from build123d import *

# Parameters (mm, degrees)
SKETCH_1_W          = 10
SKETCH_1_H          = 10
SKETCH_1_W_2        = 8
SKETCH_1_H_2        = 8
EXTRUDE_1_DEPTH     = 90
SKETCH_2_R          = 1.5
CUT_EXTRUDE_1_DEPTH = 30
SKETCH_3_R          = 1.5
CUT_EXTRUDE_2_DEPTH = 30


with BuildPart() as part:
    # 草图1 → 凸台-拉伸1 (new body)
    with BuildSketch(Plane(origin=(0, 0, 0), x_dir=(1, 0, 0), z_dir=(0, 1, 0))):
        Rectangle(SKETCH_1_W, SKETCH_1_H)
        Rectangle(SKETCH_1_W_2, SKETCH_1_H_2, mode=Mode.SUBTRACT)
    extrude(amount=EXTRUDE_1_DEPTH)

    # 草图2 → 切除-拉伸1 (cut)
    with BuildSketch(Plane.ZY.offset(5)):
        with Locations((0, 84)):
            Circle(SKETCH_2_R)
        with Locations((0, 74)):
            Circle(SKETCH_2_R)
    extrude(amount=-CUT_EXTRUDE_1_DEPTH, mode=Mode.SUBTRACT)

    # 草图3 → 切除-拉伸2 (cut)
    with BuildSketch(Plane.XY.offset(5)):
        with Locations((0, 5)):
            Circle(SKETCH_3_R)
        with Locations((0, 15)):
            Circle(SKETCH_3_R)
    extrude(amount=-CUT_EXTRUDE_2_DEPTH, mode=Mode.SUBTRACT)


solid = part.part
Read the model definition and answer for the solid it produces. Units are mm, in the model's axes. A direction names the side the tool comes from. Coordinates: 2 decimals unless noted, no trailing zeros. Loops run counter-clockwise (first coordinate to the right, second up) from the corner with the lowest first, then second, coordinate; pieces in that order, holes last. Notation, with made-up numbers: (41.5, 21.5) - (63.5, 21.5) arc R29 cw to (63.5, 43.5) - close; hole circle Ø4 at (35.25, -37). An arc over 180 degrees is marked (long way). Answer in a Markdown table with one row per item.
Q1. Find section B-B on y = 15. Write down the section's boundary in (x, z).
Here are the results:
| item | result |
|---|---|
| outline | (-5, -5) - (-1.5, -5) - (-1.5, -4) - (-4, -4) - (-4, 4) - (-1.5, 4) - (-1.5, 5) - (-5, 5) - close; (1.5, -5) - (5, -5) - (5, 5) - (1.5, 5) - (1.5, 4) - (4, 4) - (4, -4) - (1.5, -4) - close |
Q2. Straight lines are drawn through the part: line 1 along Y through (x, z) = (0, -4.2); line 2 along Y through (x, z) = (-4.3, 0); line 3 along X through (y, z) = (15.5, 1.5). For each, find the intervals that lie inside material, in ascending order. Write a range as [from, to].
Here are the results:
| item | result |
|---|---|
| line 1 | y = [0, 3.5], [6.5, 13.5], [16.5, 90] |
| line 2 | y = [0, 72.5], [75.5, 82.5], [85.5, 90] |
| line 3 | x = [-5, -4], [4, 5] |
Q3. Find section D-D on x = 0.75. Write down the section's boundary in (y, z), plus the area to 3 significant figures.
Here are the results:
| item | result |
|---|---|
| outline | (0, -5) - (3.7, -5) - (3.7, -4) - (0, -4) - close; (0, 4) - (3.7, 4) - (3.7, 5) - (0, 5) - close; (6.3, -5) - (13.7, -5) - (13.7, -4) - (6.3, -4) - close; (6.3, 4) - (13.7, 4) - (13.7, 5) - (6.3, 5) - close; (16.3, -5) - (90, -5) - (90, -4) - (16.3, -4) - close; (16.3, 4) - (90, 4) - (90, 5) - (16.3, 5) - close |
| area | 170 mm^2 |
Q4. For faces 1 (the cylindrical face through (4.493, 75.265, 0.806)), 2 (the flat face through (4, 44, 0)), determine the directions among +Z, -Z, +X, -X, +Y, -Y from which every point of the face is accessible in a straight line to the end or side of a thin tool.
Here are the results:
| item | result |
|---|---|
| face 1 | +X, -X |
| face 2 | +Y, -Y |
Q5. Given P1, Ø2.5, axis at y = 74, z = 0, coming from the +X side, flat-ended and moving along its own axis, determine where the tip first touches the part or whether it passes through.
Here are the results:
| item | result |
|---|---|
| P1 | passes through |
Q6. Find section A-A on z = 0. Write down the section's boundary in (x, y), plus the area to 3 significant figures.
Here are the results:
| item | result |
|---|---|
| outline | (-5, 0) - (-4, 0) - (-4, 72.5) - (-5, 72.5) - close; (-5, 75.5) - (-4, 75.5) - (-4, 82.5) - (-5, 82.5) - close; (-5, 85.5) - (-4, 85.5) - (-4, 90) - (-5, 90) - close; (4, 0) - (5, 0) - (5, 72.5) - (4, 72.5) - close; (4, 75.5) - (5, 75.5) - (5, 82.5) - (4, 82.5) - close; (4, 85.5) - (5, 85.5) - (5, 90) - (4, 90) - close |
| area | 168 mm^2 |
Q7. The mould has two halves that part along Y. Classify faces 3 (the flat face through (-4.5, 90, -0.1)), 4 (the cylindrical face through (-1.5, 5.07, -4.49)), 5 (the cylindrical face through (-1.11, 16.01, -4.49)), 6 (the flat face through (0, 44, 4)): pulls with the +Y half, pulls with the -Y half, needs draft (parallel to the pull), parting line crosses it, or undercut.
Here are the results:
| item | result |
|---|---|
| face 3 | pulls with the +Y half |
| face 4 | undercut |
| face 5 | undercut |
| face 6 | needs draft |
Q8. Find section C-C on y = 57.5. Write down the section's boundary in (x, z), plus the area to 3 significant figures.
Here are the results:
| item | result |
|---|---|
| outline | (-5, -5) - (5, -5) - (5, 5) - (-5, 5) - close; hole (-4, -4) - (4, -4) - (4, 4) - (-4, 4) - close |
| area | 36.0 mm^2 |
